Input: part model. Units: mm. Frame: model coordinates. Round coordinates to 2 decimals unless told otherwise and drop trailing zeros. Loops run counter-clockwise (first coordinate to the right, second up) from the corner with the lowest first, then second, coordinate; pieces in that order, holes last. Notation, with made-up numbers: M -2,17.5 L 36,17.5 A10 cw 36,30.5 Z; hole C 33,57.5 d1. An arc over 180 degrees is marked long. Return JSON: item names as keys, results as strings. Group by question number.
1) Section C-C (y = -27). Output: boundary loops of the cut face in (x, z).
2) Section B-B (y = -78.5). Output: boundary loops of the cut face in (x, z), plus the area to 3 significant figures.
3) Material intervals for line 1 (Z direction, x = 0, y = -79.5); line 2 (Y direction, x = -2.25, z = 1.5); line 3 (Y direction, x = 0, z = -0.25), sorted ascending. Write a range as from..to.
4) Contact query for flat-ended pins moving along their axis: P1, Ø2, axis at x = -2, z = -2.5, coming from the -Y side; P2, Ø1.8, axis at x = 0, z = 1, coming from the -Y side; P3, Ø3, axis at y = -41, z = -0.5, coming from the -X side; P4, Ø1.5, axis at x = -3.5, y = -64.5, coming from the -Z side. Output: stop coordinate, or through.
5) Section A-A (y = 0). Output: boundary loops of the cut face in (x, z), plus the area to 3 significant figures.
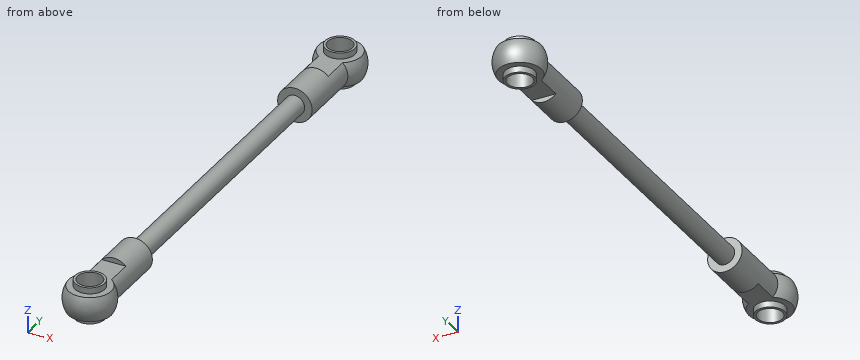
from build123d import *

# Parameters (mm, degrees)
SKETCH2_R               = 2.5
CUT_EXTRUDE1_DEPTH      = 6
CUT_EXTRUDE1_DEPTH_BACK = 6
SKETCH4_W               = 12
SKETCH4_H               = 18
CUT_EXTRUDE2_DEPTH      = 1.830127
SKETCH3_R               = 3
SKETCH3_R_2             = 2.5
EXTRUDE_THIN1_DEPTH     = 3.75
SKETCH5_R               = 2
BOSS_EXTRUDE1_DEPTH     = 30


with BuildPart() as part:
    # Sketch1 → Revolve1 (revolve)
    with BuildSketch(Plane.XY):
        with BuildLine():
            Line((0, 0), (0, -7))
            Line((0, -7), (1.75, -7))
            Line((1.75, -7), (1.75, -17))
            Line((1.75, -17), (3.5, -17))
            Line((3.5, -17), (3.5, -3.570714214))
            ThreePointArc((3.5, -3.570714214), (4.628907596, 1.890294809), (0, 5))
            Line((0, 5), (0, 0))
        make_face()
    revolve(axis=Axis((0, 0, 0), (0, 1, 0)))

    # Sketch2 → Cut-Extrude1 (cut, two sides)
    with BuildSketch(Plane.XY) as cut_extrude1_sk:
        Circle(SKETCH2_R)
    extrude(amount=CUT_EXTRUDE1_DEPTH, mode=Mode.SUBTRACT)
    extrude(cut_extrude1_sk.sketch, amount=-CUT_EXTRUDE1_DEPTH_BACK, mode=Mode.SUBTRACT)

    # Sketch4 → Cut-Extrude2 (cut)
    with BuildSketch(Plane.XY.offset(2.5)):
        Rectangle(SKETCH4_W, SKETCH4_H)
    cut_extrude2 = extrude(amount=CUT_EXTRUDE2_DEPTH, mode=Mode.SUBTRACT)

    # Mirror1: Cut-Extrude2 across plane
    add(cut_extrude2.mirror(Plane.XY), mode=Mode.SUBTRACT)

    # Sketch3 → Extrude-Thin1 (add, symmetric)
    with BuildSketch(Plane.XY):
        Circle(SKETCH3_R)
        Circle(SKETCH3_R_2, mode=Mode.SUBTRACT)
    extrude(amount=EXTRUDE_THIN1_DEPTH, both=True)


with BuildPart() as body_2:
    # Mirror3: mirrored copy
    add(part.part.mirror(Plane(origin=(0, -47, 0), x_dir=(0, 0, 1), z_dir=(0, -1, 0))))


with BuildPart() as part_1:
    add(part.part)

    add(body_2.part)  # Boss-Extrude1 merges body 2
    # Sketch5 → Boss-Extrude1 (add, symmetric)
    with BuildSketch(Plane(origin=(0, -47, 0), x_dir=(-1, 0, 0), z_dir=(0, -1, 0))):
        Circle(SKETCH5_R)
    extrude(amount=BOSS_EXTRUDE1_DEPTH, both=True)


solid = part_1.part
Returned:
{
 "1": {"outline": "C 0,0 d4"},
 "2": {"outline": "C 0,0 d7; hole C 0,0 d3.5", "area": "28.9 mm^2"},
 "3": {"line 1": "z = -3.5..-1.75, 1.75..3.5", "line 2": "y = -98.21..-95.09, -92.91..-77, -17..-1.09, 1.09..4.21", "line 3": "y = -98.99..-96.5, -91.5..-87, -77..-17, -7..-2.5, 2.5..4.99"},
 "4": {"P1": "stops at y = -98.49", "P2": "stops at y = -99", "P3": "stops at x = -2", "P4": "passes through"},
 "5": {"outline": "M -4.33,-2.5 L -3,-2.5 L -3,-3.75 L -2.5,-3.75 L -2.5,3.75 L -3,3.75 L -3,2.5 L -4.33,2.5 A5 ccw Z; M 2.5,-3.75 L 3,-3.75 L 3,-2.5 L 4.33,-2.5 A5 ccw 4.33,2.5 L 3,2.5 L 3,3.75 L 2.5,3.75 Z", "area": "25.3 mm^2"}
}
